CAD build for the part. Positions are in the model's coordinates, mm. Face numbers are marked on the shaded views. A direction names the side the tool comes from. Give positions to 0.01 mm unless a question says otherwise; leave off trailing zeros. Order: outer loops, then holes, each group sorted by start corner. A loop starts at its lowest first (then second) coordinate and runs counter-clockwise, first axis right, second up.
Item 1: Band-saw the part on A-A on y = 14.5. Give the cut face in (x, z), plus the area to 3 significant figures.
Item 2: Which spindle directions (+Z, -Z, +X, -X, +Y, -Y) get a long thin tool onto all of the face, cutting with end or side? Do the marked faces 1, 2 and 3. Say none if no direction does.
Item 3: Band-saw the part on D-D on z = -3.75. Give the cut face in (x, y).
Item 4: Band-saw the part on C-C on z = -10.5. Give the cut face in (x, y).
Item 5: Two-plate mould, pull along Y, no slides. Class the marked faces 4, 5 and 6: released by +Y, released by -Y, zero draft, split by the parting line, or undercut.
Item 6: Band-saw the part on B-B on x = 22. Give the cut face in (y, z).
Item 7: Flat gauge pins, fed straight in: P1, Ø2, axis at x = 30.5, y = 23, coming from the -Z side; P2, Ø2.5, axis at x = 18.23, y = 11.13, coming from the +Z side; P3, Ø3, axis at x = 34.5, z = 0.5, coming from the -Y side; P4, Ø3, axis at x = 34.5, y = -6, coming from the +Z side. Where does each tip first touch, or does it go through?
Item 8: Wall check: L1, parallel to X at y = 15.5, z = 0.5; L2, parallel to X at y = 24, z = 0.25; L3, parallel to Y at x = 29, z = -2.75. Give the ranges that are in metal, low to high.
```python
from build123d import *

# Parameters (mm, degrees)
SKETCH_1_W               = 40
SKETCH_1_H               = 40
EXTRUDE_1_DEPTH          = 12.7
CUT_EXTRUDE_2_DEPTH      = 0.7
CUT_EXTRUDE_2_DEPTH_BACK = 1.5
SKETCH_8_W               = 36.4
SKETCH_8_H               = 28.4
CUT_EXTRUDE_4_DEPTH      = 12.7
SKETCH_10_R              = 0.5
SKETCH_10_R_2            = 1.5
SKETCH_10_W              = 3
SKETCH_10_H              = 13
EXTRUDE_2_DEPTH          = 2.2
CUT_EXTRUDE_START        = -12.7
SKETCH_13_R              = 1.35
CUT_EXTRUDE_6_DEPTH      = 12.7
FILLET_1_R               = 1
SKETCH_14_W              = 8.31999735
SKETCH_14_H              = 2.64999918
CUT_EXTRUDE_8_DEPTH      = 5.8
SKETCH_15_W              = 12.8999835
SKETCH_15_H              = 7.3
CUT_EXTRUDE_9_DEPTH      = 5.8
SKETCH_16_W              = 1.085536683
SKETCH_16_H              = 5.100270408
CUT_EXTRUDE_10_DEPTH     = 1.8
SKETCH_17_W              = 8.31999735
SKETCH_17_H              = 2.65925193
CUT_EXTRUDE_11_DEPTH     = 5.8
SKETCH_23_W              = 6.0022214
SKETCH_23_H              = 5.598076211
SKETCH_23_H_2            = 5.598076212
CUT_EXTRUDE_12_DEPTH     = 4
SKETCH_24_W              = 11
SKETCH_24_H              = 14
CUT_EXTRUDE_14_DEPTH     = 1.4
SKETCH_22_W              = 1
SKETCH_22_H              = 0.8


with BuildPart() as part:
    # 草图1 → 凸台-拉伸1 (new body)
    with BuildSketch(Plane(origin=(0, 0, -12.4), x_dir=(-1, 0, 0), z_dir=(0, 0, -1))):
        with Locations((-18.22949197, 11.132690632)):
            Rectangle(SKETCH_1_W, SKETCH_1_H)
    extrude(amount=-EXTRUDE_1_DEPTH)

    # 草图2 → 切除-拉伸2 (cut, two sides: drawn at the far end of the back side and taken through both)
    with BuildSketch(Plane.XY.offset(-8).offset(-CUT_EXTRUDE_2_DEPTH_BACK)):
        Polygon((-2.01828663, -8.469233156), (2.73171337, -8.469233156), (4.23171337, -5.871156945), (2.72949197, -3.269233156), (-2.01828663, -3.269233156), align=None)
        Polygon((-2.01828663, 25.534614421), (-2.01828663, 30.734614421), (2.73171337, 30.734614421), (4.23171337, 28.13653821), (2.72949197, 25.534614421), align=None)
        Polygon((38.47727057, 30.734614421), (33.72727057, 30.734614421), (32.22727057, 28.13653821), (33.72949197, 25.534614421), (38.47727057, 25.534614421), align=None)
        Polygon((38.47727057, -3.269233156), (38.47727057, -8.469233156), (33.72727057, -8.469233156), (32.22727057, -5.871156945), (33.72949197, -3.269233156), align=None)
    extrude(amount=CUT_EXTRUDE_2_DEPTH + CUT_EXTRUDE_2_DEPTH_BACK, mode=Mode.SUBTRACT)

    # 草图8 → 切除-拉伸4 (cut)
    with BuildSketch(Plane(origin=(0, 0, -12.4), x_dir=(-1, 0, 0), z_dir=(0, 0, -1))):
        with Locations((-18.22949197, 11.132690632)):
            Rectangle(SKETCH_8_W, SKETCH_8_H)
    extrude(amount=-CUT_EXTRUDE_4_DEPTH, mode=Mode.SUBTRACT)

    # 草图13 → 切除-拉伸6 (cut)
    with BuildSketch(Plane(origin=(0, 0, -12.4), x_dir=(-1, 0, 0), z_dir=(0, 0, -1)).offset(CUT_EXTRUDE_START)):
        with Locations((-35.22949197, -5.867309368)):
            Circle(SKETCH_13_R)
        with Locations(Location((-1.22949197, -5.867309368, 0), (0, 0, 180))):
            Circle(SKETCH_13_R)
        with Locations((-1.22949197, 28.132690632)):
            Circle(SKETCH_13_R)
        with Locations(Location((-35.22949197, 28.132690632, 0), (0, 0, 180))):
            Circle(SKETCH_13_R)
    extrude(amount=CUT_EXTRUDE_6_DEPTH, mode=Mode.SUBTRACT)

    # 圆角1
    fillet_1_edges = [part.edges().sort_by_distance(p)[0] for p in [
        (0.02949197, 25.332690632, -6.05),
        (0.02949197, -3.067309368, -6.05),
        (36.42949197, -3.067309368, -6.05),
        (36.42949197, 25.332690632, -6.05),
    ]]
    fillet(fillet_1_edges, radius=FILLET_1_R)

    # 草图14 → 切除-拉伸8 (cut)
    with BuildSketch(Plane.XZ.offset(8.867309368)):
        with Locations((8.169941285, -11.07500041)):
            Rectangle(SKETCH_14_W, SKETCH_14_H)
    extrude(amount=-CUT_EXTRUDE_8_DEPTH, mode=Mode.SUBTRACT)

    # 草图15 → 切除-拉伸9 (cut)
    with BuildSketch(Plane.XZ.offset(8.867309368)):
        with Locations((23.79587104, -8.75)):
            Rectangle(SKETCH_15_W, SKETCH_15_H)
    extrude(amount=-CUT_EXTRUDE_9_DEPTH, mode=Mode.SUBTRACT)

    # 草图16 → 切除-拉伸10 (cut)
    with BuildSketch(Plane(origin=(38.22949197, 0, 0), x_dir=(0, 0, -1), z_dir=(1, 0, 0))):
        with Locations((11.857231659, 0.566559812)):
            Rectangle(SKETCH_16_W, SKETCH_16_H)
    extrude(amount=-CUT_EXTRUDE_10_DEPTH, mode=Mode.SUBTRACT)

    # 草图17 → 切除-拉伸11 (cut)
    with BuildSketch(Plane(origin=(0, 31.132690632, 0), x_dir=(1, 0, 0), z_dir=(0, 1, 0))):
        with Locations((28.372981895, 11.070374035)):
            Rectangle(SKETCH_17_W, SKETCH_17_H)
    extrude(amount=-CUT_EXTRUDE_11_DEPTH, mode=Mode.SUBTRACT)

    # 草图23 → 切除-拉伸12 (cut)
    with BuildSketch(Plane.XY.offset(2.5)):
        with Locations((35.22838127, 28.333652527)):
            Rectangle(SKETCH_23_W, SKETCH_23_H)
        with Locations((35.22838127, -6.068271262)):
            Rectangle(SKETCH_23_W, SKETCH_23_H_2)
        with Locations((1.23060267, -6.068271262)):
            Rectangle(SKETCH_23_W, SKETCH_23_H_2)
        with Locations((1.23060267, 28.333652527)):
            Rectangle(SKETCH_23_W, SKETCH_23_H)
    extrude(amount=-CUT_EXTRUDE_12_DEPTH, mode=Mode.SUBTRACT)


with BuildPart() as body_2:
    # 草图10 → 凸台-拉伸2 (new body)
    with BuildSketch(Plane.XY.offset(0.3)):
        Polygon((-1.77050803, 25.534614421), (4.23171337, 25.534614421), (4.23171337, 31.132690632), (32.22727057, 31.132690632), (32.22727057, 25.534614421), (38.22949197, 25.534614421), (38.22949197, -3.269233156), (32.22727057, -3.269233156), (32.22727057, -8.867309368), (4.23171337, -8.867309368), (4.23171337, -3.269233156), (-1.77050803, -3.269233156), align=None)
        with Locations((18.22949197, 11.132690632)):
            Circle(SKETCH_10_R, mode=Mode.SUBTRACT)
        with Locations((3.22949197, 0.632690632)):
            Circle(SKETCH_10_R_2, mode=Mode.SUBTRACT)
        with Locations((3.22949197, 21.632690632)):
            Circle(SKETCH_10_R_2, mode=Mode.SUBTRACT)
        with Locations(Location((33.22949197, 21.632690632, 0), (0, 0, 180))):
            Circle(SKETCH_10_R_2, mode=Mode.SUBTRACT)
        with Locations(Location((33.22949197, 0.632690632, 0), (0, 0, 180))):
            Circle(SKETCH_10_R_2, mode=Mode.SUBTRACT)
        with Locations((3.22949197, 11.132690632)):
            Rectangle(SKETCH_10_W, SKETCH_10_H, mode=Mode.SUBTRACT)
        with Locations((33.22949197, 11.132690632)):
            Rectangle(SKETCH_10_W, SKETCH_10_H, mode=Mode.SUBTRACT)
    extrude(amount=EXTRUDE_2_DEPTH)

    # 草图24 → 切除-拉伸14 (cut)
    with BuildSketch(Plane(origin=(0, 0, 0.3), x_dir=(-1, 0, 0), z_dir=(0, 0, -1))):
        with Locations((-18.22949197, 11.132690632)):
            Rectangle(SKETCH_24_W, SKETCH_24_H)
    extrude(amount=-CUT_EXTRUDE_14_DEPTH, mode=Mode.SUBTRACT)

    # 草图22 → 切除-旋转3 (revolve, cut)
    with BuildSketch(Plane(origin=(0, 11.132690632, 0), x_dir=(-1, 0, 0), z_dir=(0, -1, 0))):
        with Locations((-18.72949197, -2.1)):
            Rectangle(SKETCH_22_W, SKETCH_22_H)
    revolve(axis=Axis((18.22949197, 11.132690632, 5.06186702), (0, 0, -1)), mode=Mode.SUBTRACT)

    # Combine 1: union part
    add(part.part)


solid = body_2.part
```
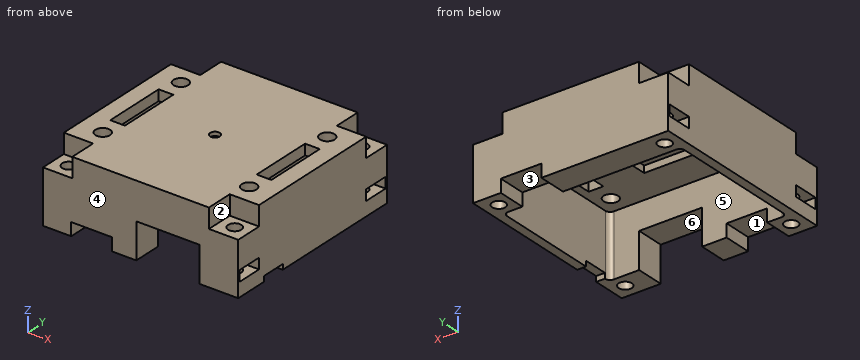
The answers:
1. outline: (-1.77, -12.4) - (0.03, -12.4) - (0.03, 0.3) - (1.73, 0.3) - (1.73, 2.5) - (-1.77, 2.5) - close; (4.73, 0.3) - (12.73, 0.3) - (12.73, 1.7) - (23.73, 1.7) - (23.73, 0.3) - (31.73, 0.3) - (31.73, 2.5) - (4.73, 2.5) - close; (34.73, 0.3) - (36.43, 0.3) - (36.43, -12.4) - (38.23, -12.4) - (38.23, 2.5) - (34.73, 2.5) - close
1. area: 105 mm2
2. face 1: -Z, -Y
2. face 2: +Z, +X, -Y
2. face 3: -Z, +Y
3. outline: (-1.77, -8.87) - (38.23, -8.87) - (38.23, 31.13) - (-1.77, 31.13) - close; hole circle Ø2.7 at (1.23, -5.87); hole circle Ø2.7 at (1.23, 28.13); hole (0.03, -2.07) arc R1 ccw to (1.03, -3.07) - (35.43, -3.07) arc R1 ccw to (36.43, -2.07) - (36.43, 24.33) arc R1 ccw to (35.43, 25.33) - (1.03, 25.33) arc R1 ccw to (0.03, 24.33) - close; hole circle Ø2.7 at (35.23, -5.87); hole circle Ø2.7 at (35.23, 28.13)
4. outline: (-1.77, -8.87) - (4.01, -8.87) - (4.01, -3.07) - (1.03, -3.07) arc R1 cw to (0.03, -2.07) - (0.03, 24.33) arc R1 cw to (1.03, 25.33) - (24.21, 25.33) - (24.21, 31.13) - (-1.77, 31.13) - close; (12.33, -8.87) - (17.35, -8.87) - (17.35, -3.07) - (12.33, -3.07) - close; (30.25, -8.87) - (38.23, -8.87) - (38.23, 31.13) - (32.53, 31.13) - (32.53, 25.33) - (35.43, 25.33) arc R1 cw to (36.43, 24.33) - (36.43, -2.07) arc R1 cw to (35.43, -3.07) - (30.25, -3.07) - close; hole circle Ø2.7 at (1.23, -5.87); hole circle Ø2.7 at (1.23, 28.13); hole circle Ø2.7 at (35.23, -5.87); hole circle Ø2.7 at (35.23, 28.13)
5. face 4: released by -Y
5. face 5: undercut
5. face 6: zero draft
6. outline: (-8.87, -5.1) - (-3.07, -5.1) - (-3.07, 0.3) - (4.13, 0.3) - (4.13, 1.7) - (18.13, 1.7) - (18.13, 0.3) - (25.33, 0.3) - (25.33, -12.4) - (31.13, -12.4) - (31.13, 2.5) - (-8.87, 2.5) - close
7. P1: stops at z = 0.3
7. P2: stops at z = 2.5
7. P3: stops at y = -3.27
7. P4: stops at z = -1.5
8. L1: x = -1.77 to 1.73, 4.73 to 12.73, 23.73 to 31.73, 34.73 to 38.23
8. L2: x = -1.77 to 0.03, 36.43 to 38.23
8. L3: y = -8.87 to -3.07, 25.33 to 31.13
